Could you check a few things on this model? Use its own coordinates, in mm. Give positions to 0.01 mm unless a question says otherwise; leave off trailing zeros. Loops run counter-clockwise (first coordinate to the right, second up) from the corner with the lowest first, then second, coordinate; pieces in that order, holes last. Notation, with made-up numbers: M -16.75,57 L 7.25,57 A29 ccw 7.25,86 Z; hole C 61,50 d9. An arc over 180 degrees is marked long. Answer in a Markdown table with one row per item. Add a question column.
```python
from build123d import *

# Parameters (mm, degrees)
F0_R     = 6
F1_DEPTH = 76.2
F3_R     = 6
F3_R_2   = 5.715
F4_DEPTH = 1.27
F5_SIZE  = 1.27


with BuildPart() as f1:
    # F0 (on Top) → F1 (new body)
    with BuildSketch(Plane.XY):
        Circle(F0_R)
    extrude(amount=F1_DEPTH)

    # F3 (on offset) → F4 (cut)
    with BuildSketch(Plane(origin=(0, 0, 6.35), x_dir=(1, 0, 0), z_dir=(0, 0, -1))):
        Circle(F3_R)
        Circle(F3_R_2, mode=Mode.SUBTRACT)
    extrude(amount=F4_DEPTH, mode=Mode.SUBTRACT)

    # F5
    f5_edges = [f1.edges().sort_by_distance(p)[0] for p in [
        (-6, 0, 0),
        (-6, 0, 76.2),
    ]]
    chamfer(f5_edges, length=F5_SIZE)


solid = f1.part
```
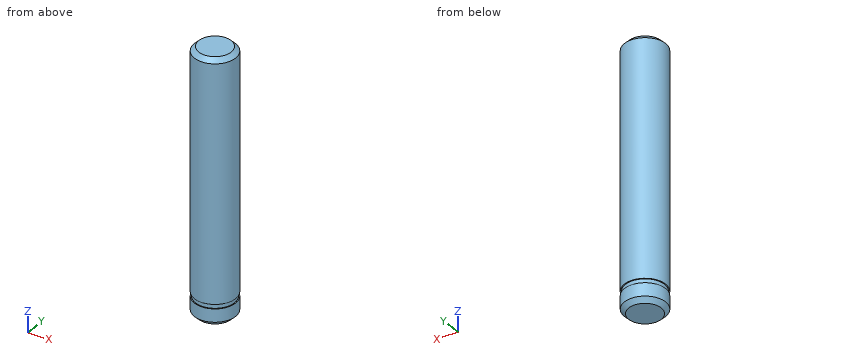
Item 1: For P1, Ø4, axis at x = 4, z = 35.5, coming from the -Y side; P2, Ø6, axis at x = -2.5, y = -3, coming from the -Z side; P3, Ø1, axis at y = 5, z = 56.5, coming from the +X side, each with a flat end and sliding along its axis, tell me the tip position at first contact or that it passes through.
Item 2: I need wall thicknesses on L1, parallel to X at y = -0.25, z = 67.5; L2, parallel to Y at x = -4, z = 27.5; L3, parallel to Y at x = -5.25, z = 34. Which ranges of each line are inside material? Lowest first, please.
Item 3: Suppose I cut it at A-A (z = 19.5). List the corners of the cut face in (x, y) for me.
Values found:
| question | item | result |
|---|---|---|
| 1 | P1 | y = -5.66 |
| 1 | P2 | z = 0 |
| 1 | P3 | x = 3.97 |
| 2 | L1 | -5.99 to 5.99 |
| 2 | L2 | -4.47 to 4.47 |
| 2 | L3 | -2.9 to 2.9 |
| 3 | outline | C 0,0 d12 |
